Geometry check sheet. Reference: the model listing, model coordinates, mm. Face numbers are marked on the shaded views. A direction names the side the tool comes from. Coordinates: 2 decimals unless noted, no trailing zeros. Loops run counter-clockwise (first coordinate to the right, second up) from the corner with the lowest first, then second, coordinate; pieces in that order, holes last.
from build123d import *

# Parameters (mm, degrees)
F0_W     = 25
F0_H     = 25
F1_DEPTH = 25.4
F2_R     = 2.5
F2_R_2   = 2.5019
F3_DEPTH = 1
F4_R     = 2.5019
F5_DEPTH = 2
F6_R     = 2.5019
F7_DEPTH = 2


with BuildPart() as f1:
    # F0 (on Front) → F1 (new body)
    with BuildSketch(Plane.XZ):
        with Locations((-12.5, 24.625)):
            Rectangle(F0_W, F0_H)
    extrude(amount=F1_DEPTH)

    # F2 (on face) → F3 (cut)
    with BuildSketch(Plane.XZ.offset(25.4)):
        with Locations((-20, 32.125)):
            Circle(F2_R)
        with Locations((-12.5, 24.625)):
            Circle(F2_R_2)
        with Locations((-5.0038, 32.1212)):
            Circle(F2_R_2)
        with Locations((-5.0038, 17.6269)):
            Circle(F2_R_2)
        with Locations((-20, 17.6269)):
            Circle(F2_R_2)
    extrude(amount=-F3_DEPTH, mode=Mode.SUBTRACT)

    # F4 (on face) → F5 (cut)
    with BuildSketch(Plane(origin=(0, 0, 0), x_dir=(-1, 0, 0), z_dir=(0, 1, 0))):
        with Locations((5.0038, 32.1212)):
            Circle(F4_R)
        with Locations((19.9962, 17.1288)):
            Circle(F4_R)
    extrude(amount=-F5_DEPTH, mode=Mode.SUBTRACT)

    # F6 (on face) → F7 (cut)
    with BuildSketch(Plane(origin=(0, 0, 12.125), x_dir=(1, 0, 0), z_dir=(0, 0, -1))):
        with Locations((-5.0038, 5.3848)):
            Circle(F6_R)
        with Locations((-20.2438, 12.8905)):
            Circle(F6_R)
        with Locations((-5.0038, 12.8905)):
            Circle(F6_R)
        with Locations((-5.0038, 20.3962)):
            Circle(F6_R)
        with Locations((-20.2438, 20.3962)):
            Circle(F6_R)
        with Locations((-20.2438, 5.3848)):
            Circle(F6_R)
    extrude(amount=-F7_DEPTH, mode=Mode.SUBTRACT)


solid = f1.part
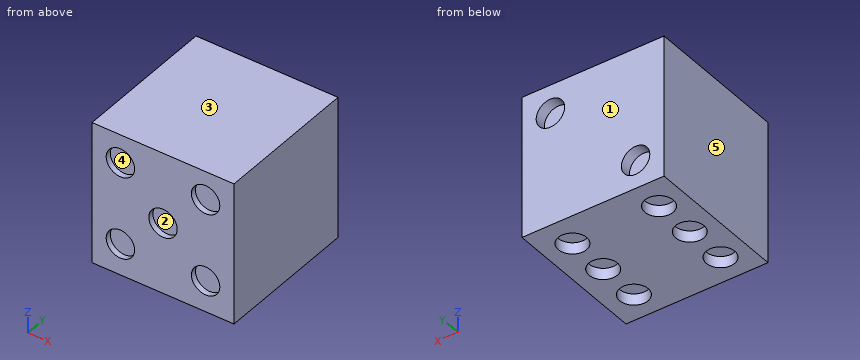
1) Section check D-D on z = 33.75. Record the cut outline in (x, y), and give its area (3 significant figures).
Data:
outline: (-25, -25.4) - (-21.9, -25.4) - (-21.9, -24.4) - (-18.1, -24.4) - (-18.1, -25.4) - (-6.9, -25.4) - (-6.9, -24.4) - (-3.1, -24.4) - (-3.1, -25.4) - (0, -25.4) - (0, 0) - (-3.1, 0) - (-3.1, -2) - (-6.9, -2) - (-6.9, 0) - (-25, 0) - close
area: 620 mm2
2) Access from +Z, -Z, +X, -X, +Y, -Y to the whole of each face (thin tool, end or side, straight path). Record for the marked faces 1 and 2.
Data:
face 1: +Z, -Z, +X, -X, +Y
face 2: -Y
3) Section check C-C on y = -18.75. Record the cut outline in (x, z) (3 decimals).
Data:
outline: (-25, 12.125) - (-22.128, 12.125) - (-22.128, 14.125) - (-18.36, 14.125) - (-18.36, 12.125) - (-6.888, 12.125) - (-6.888, 14.125) - (-3.12, 14.125) - (-3.12, 12.125) - (0, 12.125) - (0, 37.125) - (-25, 37.125) - close
4) Mould release check, pull along Z, two halves, no side actions. Record for the marked faces 3, 4 and 5: +Z half, -Z half, draft (parallel to the pull), parting line (faces both ways), or undercut.
Data:
face 3: +Z half
face 4: undercut
face 5: draft
5) Material ranges on probe 1 along Z at (x, y) = (-20.5, -21) (3 decimals); probe 2 along Y at (x, z) = (-4.5, 15.5); probe 3 along Y at (x, z) = (-3.25, 32.5), recorded low to high.
Data:
probe 1: z = 14.125 to 37.125
probe 2: y = -24.4 to 0
probe 3: y = -24.4 to -2
6) Section check A-A on x = -19.25. Record the cut outline in (y, z) (3 decimals), and give its area (3 significant figures).
Data:
outline: (-25.4, 12.125) - (-22.692, 12.125) - (-22.692, 14.125) - (-18.1, 14.125) - (-18.1, 12.125) - (-15.187, 12.125) - (-15.187, 14.125) - (-10.594, 14.125) - (-10.594, 12.125) - (-7.681, 12.125) - (-7.681, 14.125) - (-3.089, 14.125) - (-3.089, 12.125) - (0, 12.125) - (0, 14.741) - (-2, 14.741) - (-2, 19.517) - (0, 19.517) - (0, 37.125) - (-25.4, 37.125) - (-25.4, 34.51) - (-24.4, 34.51) - (-24.4, 29.74) - (-25.4, 29.74) - (-25.4, 20.014) - (-24.4, 20.014) - (-24.4, 15.24) - (-25.4, 15.24) - close
area: 588 mm2
7) Depth check by flat-ended pin: pin 1 (3 mm diameter, centred on x = -5, z = 32.12, fed in from -Y); pin 2 (1.5 mm diameter, centred on x = -5, y = -5.5, fed in from -Z) (3 decimals). Enter the tip coordinate at first touch or a pass-through.
Data:
pin 1: stops at y = -24.4
pin 2: stops at z = 14.125
8) Section check B-B on z = 30. Record the cut outline in (x, y), and give its area (3 significant figures).
Data:
outline: (-25, -25.4) - (-21.32, -25.4) - (-21.32, -24.4) - (-18.68, -24.4) - (-18.68, -25.4) - (-6.33, -25.4) - (-6.33, -24.4) - (-3.68, -24.4) - (-3.68, -25.4) - (0, -25.4) - (0, 0) - (-3.68, 0) - (-3.68, -2) - (-6.33, -2) - (-6.33, 0) - (-25, 0) - close
area: 624 mm2
